```python
from build123d import *

# Parameters (mm, degrees)
SKETCH1_R           = 6.1
SKETCH1_R_2         = 1.5
BOSS_EXTRUDE1_DEPTH = 2.3
SKETCH2_R           = 4.4
SKETCH2_R_2         = 3
BOSS_EXTRUDE2_DEPTH = 3.2
SKETCH3_R           = 0.75
BOSS_EXTRUDE3_DEPTH = 2.3
CIRPATTERN1_COUNT   = 2


with BuildPart() as part:
    # Sketch1 → Boss-Extrude1 (new body)
    with BuildSketch(Plane(origin=(0, 0, 0), x_dir=(1, 0, 0), z_dir=(0, 1, 0))):
        Circle(SKETCH1_R)
        Circle(SKETCH1_R_2, mode=Mode.SUBTRACT)
    extrude(amount=BOSS_EXTRUDE1_DEPTH)

    # Sketch2 → Boss-Extrude2 (add)
    with BuildSketch(Plane(origin=(0, 2.3, 0), x_dir=(1, 0, 0), z_dir=(0, 1, 0))):
        Circle(SKETCH2_R)
        Circle(SKETCH2_R_2, mode=Mode.SUBTRACT)
    extrude(amount=BOSS_EXTRUDE2_DEPTH)

    # Sketch3 → Boss-Extrude3 (add)
    with BuildSketch(Plane.XZ):
        with BuildLine():
            Line((-4.5, -4.118252056), (-2.468988638, -16.892549493))
            ThreePointArc((-2.468988638, -16.892549493), (0, -19), (2.468988638, -16.892549493))
            Line((2.468988638, -16.892549493), (4.5, -4.118252056))
            ThreePointArc((4.5, -4.118252056), (0, -6.1), (-4.5, -4.118252056))
        make_face()
        with Locations((0, -16)):
            Circle(SKETCH3_R, mode=Mode.SUBTRACT)
        with Locations((0, -13)):
            Circle(SKETCH3_R, mode=Mode.SUBTRACT)
        with Locations((0, -10)):
            Circle(SKETCH3_R, mode=Mode.SUBTRACT)
        with Locations((0, -7)):
            Circle(SKETCH3_R, mode=Mode.SUBTRACT)
    boss_extrude3 = extrude(amount=-BOSS_EXTRUDE3_DEPTH)

    # CirPattern1: Boss-Extrude3 ×2 about axis
    cirpattern1_axis = Axis((0, 0, 0), (0, 1, 0))
    for i in range(1, CIRPATTERN1_COUNT):
        add(boss_extrude3.rotate(cirpattern1_axis, i * 360 / CIRPATTERN1_COUNT))


solid = part.part
```
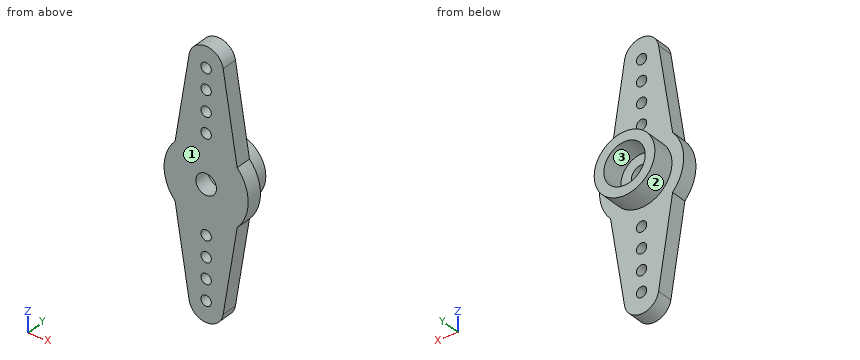
Geometry check sheet. Reference: the model listing, model coordinates, mm. Face numbers are marked on the shaded views. Coordinates: 2 decimals unless noted, no trailing zeros. Loops run counter-clockwise (first coordinate to the right, second up) from the corner with the lowest first, then second, coordinate; pieces in that order, holes last. Notation, with made-up numbers: (28, -29.5) - (45, -29.5) arc R31 cw to (45, -5.5) - close; hole circle Ø3 at (-3.75, -35). An arc over 180 degrees is marked (long way). One line per item, written item: value. Start each with the question number.
(1) Material ranges on line 1 (X direction, y = 4.3, z = 0); line 2 (Y direction, x = 2.75, z = -4); line 3 (X direction, y = 0.6, z = 7), recorded low to high. Write a range as [from, to].
(2) Mould release check, pull along X, two halves, no side actions. Record for the marked faces 1, 2 and 3: released by +X, released by -X, zero draft, split by the parting line, or undercut.
(3) Cross-section at B-B on y = 0.6. Count the separate pieces of the cut face and the enclosed holes in it, plus the area to 3 significant figures.
(4) Cross-section at C-C on x = -4. Enter the section's corners in (y, z).
(5) Depth check by flat-ended pin: P1, Ø1.2, axis at x = 0, z = -13, coming from the -Y side; P2, Ø2, axis at y = 2, z = -6, coming from the -X side; P3, Ø1, axis at y = 1.5, z = -14, coming from the -X side; P4, Ø3.5, axis at x = 0, z = 0, coming from the +Y side. Enter the tip coordinate at first touch or a pass-through.
(6) Cross-section at D-D on z = 16. Enter the section's corners in (x, y).
(7) Cross-section at A-A on z = 0. Enter the section's corners in (x, y).
Results below:
1. line 1: x = [-4.4, -3], [3, 4.4]
1. line 2: y = [0, 2.3]
1. line 3: x = [-4.04, -0.75], [0.75, 4.04]
2. face 1: zero draft
2. face 2: split by the parting line
2. face 3: undercut
3. separate pieces: 1
3. enclosed holes: 9
3. area: 265 mm2
4. outline: (0, -7.26) - (2.3, -7.26) - (2.3, -1.83) - (5.5, -1.83) - (5.5, 1.83) - (2.3, 1.83) - (2.3, 7.26) - (0, 7.26) - close
5. P1: passes through
5. P2: stops at x = -4.36
5. P3: stops at x = -3.01
5. P4: stops at y = 2.3
6. outline: (-2.61, 0) - (-0.75, 0) - (-0.75, 2.3) - (-2.61, 2.3) - close; (0.75, 0) - (2.61, 0) - (2.61, 2.3) - (0.75, 2.3) - close
7. outline: (-6.1, 0) - (-1.5, 0) - (-1.5, 2.3) - (-3, 2.3) - (-3, 5.5) - (-4.4, 5.5) - (-4.4, 2.3) - (-6.1, 2.3) - close; (1.5, 0) - (6.1, 0) - (6.1, 2.3) - (4.4, 2.3) - (4.4, 5.5) - (3, 5.5) - (3, 2.3) - (1.5, 2.3) - close
